Geometry check sheet. Reference: the model listing, model coordinates, mm. A direction names the side the tool comes from. Round coordinates to 2 decimals unless told otherwise and drop trailing zeros. Write each loop counter-clockwise with the first axis right and the second up, starting at its lowest first coordinate (ties: lowest second). Pieces come first, ordered by that corner, then holes. Notation, with made-up numbers: (-9, -2) -> (-5, -2) arc R10 ccw to (-5, 3) -> close; hole circle Ø8 at (45.5, 3.5). An arc over 180 degrees is marked (long way). Put each result on its own line as item: value. Start each with the question number.
from build123d import *

# Parameters (mm, degrees)
SALIENTE_EXTRUIR1_DEPTH = 25
CORTAR_EXTRUIR1_DEPTH   = 25


with BuildPart() as part:
    # Croquis1 → Saliente-Extruir1 (new body)
    with BuildSketch(Plane.XY):
        with BuildLine():
            Line((0, 16), (0, 15.25))
            ThreePointArc((0, 15.25), (-15.25, 0), (0, -15.25))
            Line((0, -15.25), (0, -16))
            ThreePointArc((0, -16), (-16, 0), (0, 16))
        make_face()
    extrude(amount=SALIENTE_EXTRUIR1_DEPTH)

    # Croquis2 → Cortar-Extruir1 (cut)
    with BuildSketch(Plane(origin=(0, 0, 0), x_dir=(1, 0, 0), z_dir=(0, 1, 0))):
        with BuildLine():
            Line((-4, -7), (-4, -18))
            ThreePointArc((-4, -18), (-5, -19), (-6, -18))
            Line((-6, -18), (-6, -7))
            ThreePointArc((-6, -7), (-5, -6), (-4, -7))
        make_face()
    extrude(amount=-CORTAR_EXTRUIR1_DEPTH, mode=Mode.SUBTRACT)


solid = part.part
(1) Mould release check, pull along Z, two halves, no side actions. Record for faces 3 (the flat face through (-6, -14.4, 12.6)), 4 (the flat face through (-15.7, 0.1, 25)), 5 (the flat face through (-15.7, 0.1, 0)): +Z half, -Z half, draft (parallel to the pull), parting line (faces both ways), or undercut.
(2) Sectioned sample at A-A (z = 14.5). Record the cut outline in (x, y), and give its area (3 significant figures).
(3) Go/stop test with flat-tipped pins: pin 1 Ø2 at (x, z) = (-10.5, 6.5) entering from -Y; pin 2 Ø8 at (x, z) = (-13, 6.5) entering from +Y; pin 3 Ø8 at (x, z) = (-10.5, 4) entering from +Y. Record where each tip stops, or that it passes through.
(4) Material ranges on L1, parallel to Y at x = -3.5, z = 8.75; L2, parallel to Y at x = -13, z = 5.5; L3, parallel to X at y = -5, z = 1.5, recorded low to high. Write a range as from..to.
(5) Sectioned sample at B-B (x = -2.25). Record the cut outline in (y, z).
(6) Sectioned sample at C-C (y = -6). Record the cut outline in (x, z).
(7) Sectioned sample at D-D (z = 4.5). Record the cut outline in (x, y), and give its area (3 significant figures).
(8) Set-up check for faces 1 (the cylindrical face through (-15.246, 0.335, 12.325)), 2 (the cylindrical face through (-5, -15, 19)): record each of +Z, -Z, +X, -X, +Y, -Y from which the full face is reachable in a straight line by a thin tool's end or side.
Found:
1. face 3: undercut
1. face 4: +Z half
1. face 5: -Z half
2. outline: (-6, -14.83) -> (-6, -14.02) arc R15.25 cw to (0, 15.25) -> (0, 16) arc R16 ccw to start; (-4, -15.49) arc R16 ccw to (0, -16) -> (0, -15.25) arc R15.25 cw to (-4, -14.72) -> close
2. area: 35.2 mm2
3. pin 1: y = -12.87
3. pin 2: y = 13.23
3. pin 3: y = 14.62
4. L1: -15.61..-14.84, 14.84..15.61
4. L2: -9.33..-7.97, 7.97..9.33
4. L3: -15.2..-14.41
5. outline: (-15.84, 0) -> (-15.08, 0) -> (-15.08, 25) -> (-15.84, 25) -> close; (15.08, 0) -> (15.84, 0) -> (15.84, 25) -> (15.08, 25) -> close
6. outline: (-14.83, 0) -> (-14.02, 0) -> (-14.02, 25) -> (-14.83, 25) -> close
7. outline: (0, -16) -> (0, -15.25) arc R15.25 cw to (0, 15.25) -> (0, 16) arc R16 ccw to start
7. area: 36.8 mm2
8. face 1: +Z, -Z, +X
8. face 2: -Y
